Work out the finished part from the listing and answer in its coordinate system (mm). Round coordinates to 2 decimals unless told otherwise and drop trailing zeros. Loops run counter-clockwise (first coordinate to the right, second up) from the corner with the lowest first, then second, coordinate; pieces in that order, holes last. Notation, with made-up numbers: M -0.5,15.25 L 24.5,15.25 A29 ccw 24.5,44.25 Z; hole C 19.5,-31.75 d4. An arc over 180 degrees is marked long. One line per item, written item: value.
```python
from build123d import *

# Parameters (mm, degrees)
F0_W     = 19.05
F0_H     = 19.05
F1_DEPTH = 25.4


with BuildPart() as f1:
    # F0 (on Top) → F1 (new body)
    with BuildSketch(Plane.XY):
        Rectangle(F0_W, F0_H)
    extrude(amount=-F1_DEPTH)

    # F3 (on 3pt) → F4 (revolve, cut)
    with BuildSketch(Plane(origin=(0, 0, 0), x_dir=(0.7071067812, 0.7071067812, 0), z_dir=(0.7071067812, -0.7071067812, 0))):
        with BuildLine():
            ThreePointArc((0, 3.9453841816), (9.525, 0), (13.4703841816, -9.525))
            Line((13.4703841816, -9.525), (16.0103841816, -9.525))
            Line((16.0103841816, -9.525), (16.0103841816, 6.4853841816))
            Line((16.0103841816, 6.4853841816), (0, 6.4853841816))
            Line((0, 6.4853841816), (0, 3.9453841816))
        make_face()
    revolve(axis=Axis((0, 0, -8.7556987966), (0, 0, -1)), mode=Mode.SUBTRACT)


solid = f1.part
```
1) Find the intervals of material crossed by probe 1 along X at (y, z) = (8.5, -3.25); probe 2 along Z at (x, y) = (-5.75, 7.75); probe 3 along Z at (x, y) = (-6.75, -7.5), in increasing order. Write a range as from..to.
Check values:
probe 1: -8.36..8.36
probe 2: -25.4..-0.13
probe 3: -25.4..-0.6
2) Find section A-A (z = -3). Give the vertices of the cut face in (x, y) (3 decimals), then the cut area to 3 significant figures.
Check values:
outline: M -9.525,-6.939 A11.785 ccw -6.939,-9.525 L 6.939,-9.525 A11.785 ccw 9.525,-6.939 L 9.525,6.939 A11.785 ccw 6.939,9.525 L -6.939,9.525 A11.785 ccw -9.525,6.939 Z
area: 351 mm2
3) Find section B-B (y = 7.5). Give the vertices of the cut face in (x, z) (3 decimals).
Check values:
outline: M -9.525,-25.4 L 9.525,-25.4 L 9.525,-3.653 A11.189 ccw 5.872,0 L -5.872,0 A11.189 ccw -9.525,-3.653 Z
4) This flat-tipped pin is pushed along its axis until it touches: pin 1 (4 mm diameter, centred on x = 6.5, y = 3, fed in from +Z). Where does it stop, or does it pass through?
Check values:
pin 1: z = 0
